Input: part model. Units: mm. Frame: model coordinates. A direction names the side the tool comes from. Round coordinates to 2 decimals unless told otherwise and drop trailing zeros. Write each loop counter-clockwise with the first axis right and the second up, starting at its lowest first coordinate (ties: lowest second). Pieces come first, ordered by that corner, then holes. Notation, with made-up numbers: M 84.5,-19 L 117.5,-19 A6 cw 117.5,-10 Z; hole C 45.5,17.25 d8. An arc over 180 degrees is marked long. Use one line per item in the form item = value. Start each with the question number.
```python
from build123d import *

# Parameters (mm, degrees)
BOX052_W               = 11
BOX052_H               = 11
BOX052_DEPTH           = 48
BOX052_ROLL_ANGLE      = -2.200006
BOX052_PITCH_ANGLE     = 12.000025
BOX052_PLACEMENT_ANGLE = -1e-06
BOX053_W               = 57
BOX053_H               = 5
BOX053_DEPTH           = 40
FILLET060_R            = 2.5
BOX006_W               = 11
BOX006_H               = 11
BOX006_DEPTH           = 48
BOX006_ROLL_ANGLE      = -2.200006
BOX006_PITCH_ANGLE     = 12.000025
BOX006_PLACEMENT_ANGLE = -1e-06
BOX005_W               = 58
BOX005_H               = 1
BOX005_DEPTH           = 42
FILLET058_R            = 3


with BuildPart() as cube478:
    # Box052 → Box052 (new body)
    with BuildSketch(Plane.XY):
        with Locations((5.5, 5.5)):
            Rectangle(BOX052_W, BOX052_H)
    extrude(amount=BOX052_DEPTH)


with BuildPart() as cube478_1:
    # Box052 roll: moved
    add(cube478.part.rotate(Axis((0, 0, 0), (1, 0, 0)), BOX052_ROLL_ANGLE))


with BuildPart() as cube478_2:
    # Box052 pitch: moved
    add(cube478_1.part.rotate(Axis((0, 0, 0), (0, 1, 0)), BOX052_PITCH_ANGLE))


with BuildPart() as cube478_3:
    # Box052 placement: moved
    add(cube478_2.part.moved(Location((9.5, -2, 70))).rotate(Axis((9.5, -2, 70), (0, 0, 1)), BOX052_PLACEMENT_ANGLE))


with BuildPart() as fillet060:
    # Box053 → Box053 (new body)
    with BuildSketch(Plane(origin=(19.5, 2, 71), x_dir=(1, 0, 0), z_dir=(0, 0, 1))):
        with Locations((28.5, 2.5)):
            Rectangle(BOX053_W, BOX053_H)
    extrude(amount=BOX053_DEPTH)

    # Cut038: cut Cube478
    add(cube478_3.part, mode=Mode.SUBTRACT)

    # Fillet060
    fillet060_edges = [fillet060.edges().sort_by_distance(p)[0] for p in [
        (76.5, 4.5, 71),
        (20.958305, 4.5, 71),
        (76.5, 4.5, 111),
        (29.460585, 4.5, 111),
    ]]
    fillet(fillet060_edges, radius=FILLET060_R)


with BuildPart() as cube364:
    # Box006 → Box006 (new body)
    with BuildSketch(Plane.XY):
        with Locations((5.5, 5.5)):
            Rectangle(BOX006_W, BOX006_H)
    extrude(amount=BOX006_DEPTH)


with BuildPart() as cube364_1:
    # Box006 roll: moved
    add(cube364.part.rotate(Axis((0, 0, 0), (1, 0, 0)), BOX006_ROLL_ANGLE))


with BuildPart() as cube364_2:
    # Box006 pitch: moved
    add(cube364_1.part.rotate(Axis((0, 0, 0), (0, 1, 0)), BOX006_PITCH_ANGLE))


with BuildPart() as cube364_3:
    # Box006 placement: moved
    add(cube364_2.part.moved(Location((8.5, -2, 70))).rotate(Axis((8.5, -2, 70), (0, 0, 1)), BOX006_PLACEMENT_ANGLE))


with BuildPart() as cut039:
    # Box005 → Box005 (new body)
    with BuildSketch(Plane(origin=(19.5, 2, 70), x_dir=(1, 0, 0), z_dir=(0, 0, 1))):
        with Locations((29, 0.5)):
            Rectangle(BOX005_W, BOX005_H)
    extrude(amount=BOX005_DEPTH)

    # Cut002: cut Cube364
    add(cube364_3.part, mode=Mode.SUBTRACT)

    # Fillet058
    fillet058_edges = [cut039.edges().sort_by_distance(p)[0] for p in [
        (77.5, 2.5, 70),
        (19.745748, 2.5, 70),
        (77.5, 2.5, 112),
        (28.673142, 2.5, 112),
    ]]
    fillet(fillet058_edges, radius=FILLET058_R)

    # Cut039: cut Fillet060
    add(fillet060.part, mode=Mode.SUBTRACT)


solid = cut039.part
```
Item 1: Ray query, line 1 (Z direction, x = 53.5, y = 2.55); line 2 (X direction, y = 2.85, z = 98.5); line 3 (X direction, y = 2.5, z = 96). Return the intervals inside material, ascending. Write a range as from..to.
Item 2: Reachability of faces 4 (the face through (75.748, 2.507, 71.713)), 5 (the face through (46.7, 2, 70.7)) from +Z, -Z, +X, -X, +Y, -Y: full face, straight path, thin tool, end or side. Return the list, or none.
Item 3: Cut plane A-A (x = 39). Output: boundary loops of the cut face in (y, z), plus the area to 3 significant figures.
Item 4: Cut plane C-C (z = 84.5). Output: boundary loops of the cut face in (x, y).
Item 5: Draft query along Z for faces 1 (the face through (75.787, 2.507, 110.248)), 2 (the face through (76.6, 2.51, 70.86)), 3 (the face through (29.24, 2.49, 111.35)). Return one class per face: +Z half, -Z half, draft (parallel to the pull), parting line (faces both ways), or undercut.
Item 6: Cut plane B-B (y = 2.45). Output: boundary loops of the cut face in (x, z), plus the area to 3 significant figures.
Item 7: First-contact query: pin 1 (5 mm diameter, centred on x = 68, z = 106.5, fed in from +Y). Flat tip, straight axial feed; report the tip coordinate or a pass-through.
Final values:
q1.line_1 = 70..71, 111..112
q1.line_2 = 25.8..26.8, 76.5..77.5
q1.line_3 = 25.27..26.27, 76.5..77.5
q2.face_4 = +Y, -Y
q2.face_5 = +Z, -Z, +X, -X, -Y
q3.outline = M 2,70 L 3,70 L 3,71 L 2,71 Z; M 2,111 L 3,111 L 3,112 L 2,112 Z
q3.area = 2.00 mm^2
q4.outline = M 22.83,2 L 23.83,2 L 23.83,3 L 22.83,3 Z; M 76.5,2 L 77.5,2 L 77.5,3 L 76.5,3 Z
q5.face_1 = undercut
q5.face_2 = -Z half
q5.face_3 = +Z half
q6.outline = M 20.52,73.62 A3 ccw 23.45,70 L 74.5,70 A3 ccw 77.5,73 L 77.5,109 A3 ccw 74.5,112 L 31.1,112 A3 ccw 28.17,109.62 Z; hole M 21.6,74.02 A2.5 ccw 24.05,71 L 74,71 A2.5 ccw 76.5,73.5 L 76.5,108.5 A2.5 ccw 74,111 L 31.49,111 A2.5 ccw 29.04,109.02 Z
q6.area = 184 mm^2
q7.pin_1 = through
